```python
from build123d import *

# Parameters (mm, degrees)
SKETCH_1_R      = 1
SKETCH_1_W      = 5
SKETCH_1_H      = 2.8
EXTRUDE_1_DEPTH = 1.4


with BuildPart() as part:
    # Эскиз1 → Бобышка-Вытянуть1 (new, symmetric)
    with BuildSketch(Plane.XY):
        with BuildLine():
            ThreePointArc((223.382624747, 5.634990628), (219.398084745, 3.984540168), (217.747634119, 2.35e-07))
            ThreePointArc((217.747634119, 2.35e-07), (219.398084579, -3.984540002), (223.382624747, -5.634990628))
            add(Edge.make_bspline(
                [(223.382624746, -5.634990613), (224.328656864, -5.56201019), (226.923894547, -5.35916654), (231.150377303, -5.017351086), (234.870714804, -4.704112055), (236.94221324, -4.525459463), (237.382624747, -4.487285848)],
                knots=[0.670161589, 0.670161589, 0.670161589, 0.670161589, 0.686667237, 0.715444849, 0.743923546, 0.751613474, 0.751613474, 0.751613474, 0.751613474], degree=3))
            Line((237.382624747, -4.487285848), (241.902085906, -8.639702096))
            ThreePointArc((241.902085906, -8.639702096), (243.345073916, -9.164930306), (244.73509722, -8.51230922))
            Line((244.73509722, -8.51230922), (249.382624747, -3.400128388))
            add(Edge.make_bspline(
                [(249.382624747, -3.400128388), (251.158571989, -3.232274224), (254.371192488, -2.923000161), (258.952644662, -2.467188138), (263.047743378, -2.047856604), (266.898988862, -1.642607304), (270.455833183, -1.258590905), (273.651166984, -0.905304265), (276.385426802, -0.596436482), (278.45259621, -0.358958361), (279.592043704, -0.226075898), (280, -0.1785)],
                knots=[0.821480844, 0.821480844, 0.821480844, 0.821480844, 0.852512115, 0.877624446, 0.901571134, 0.924121062, 0.944988816, 0.963803939, 0.980044339, 0.992855276, 1, 1, 1, 1], degree=3))
            ThreePointArc((280, -0.1785), (280.073937121, 0), (280, 0.1785))
            add(Edge.make_bspline(
                [(280, 0.1785), (279.592043704, 0.226075898), (278.45259621, 0.358958361), (276.385426802, 0.596436482), (273.651166984, 0.905304265), (270.455833183, 1.258590905), (266.898988862, 1.642607304), (263.047743378, 2.047856604), (258.952644662, 2.467188138), (253.116111921, 3.047869044), (247.071089236, 3.62220531), (240.854179313, 4.184912649), (236.038226964, 4.605811749), (231.150377303, 5.017351103), (226.923894547, 5.359166556), (224.328656864, 5.562010205), (223.382624747, 5.634990628)],
                knots=[0, 0, 0, 0, 0.007144724, 0.019955661, 0.036196061, 0.055011184, 0.075878938, 0.098428866, 0.122375554, 0.147487885, 0.200459747, 0.22800517, 0.256076454, 0.284555151, 0.313332763, 0.329838411, 0.329838411, 0.329838411, 0.329838411], degree=3))
        make_face()
        with Locations((243.382624747, -6.903125596)):
            Circle(SKETCH_1_R, mode=Mode.SUBTRACT)
        with Locations((223.382624747, 0)):
            Circle(SKETCH_1_R, mode=Mode.SUBTRACT)
        with Locations((243.382624747, 0)):
            Rectangle(SKETCH_1_W, SKETCH_1_H, mode=Mode.SUBTRACT)
    extrude(amount=EXTRUDE_1_DEPTH, both=True)


solid = part.part
```
Here's how the part is built. I have some questions about the finished solid (model axes, mm). A direction names the side the tool comes from. Give positions to 0.01 mm unless a question says otherwise; leave off trailing zeros. Answer as a JSON object with one key per item and string values. Group by question number.
Item 1: For P1, Ø1, axis at x = 262, z = 0, coming from the +Y side; P2, Ø0.8, axis at y = 0.5, z = -0.5, coming from the +X side; P3, Ø0.8, axis at x = 242.5, z = 0.5, coming from the +Y side, each with a flat end and sliding along its axis, tell me the tip position at first contact or that it passes through.
Item 2: If we mould it in two halves opening along Y, with no side actions, what happens to faces 1 (the flat face through (243, 1.4, 0)), 2 (the flat face through (240.883, 0, 0)), 3 (the cylindrical face through (217.75, 0.12, 0.02)), 4 (the flat face through (247.03, -5.99, 0.02))? For each: pulls with the +Y half, pulls with the -Y half, needs draft (parallel to the pull), parting line crosses it, or undercut.
Item 3: If we section it at A-A on z = -0.45: Give the number of separate pieces and of enclosed holes in the cut face, and give its area (3 significant figures).
Item 4: Please list where these lines run through material, in increasing order: probe 1 along Y at (x, z) = (223.5, 1.2); probe 2 along X at (y, z) = (-7, 0.75); probe 3 along X at (y, z) = (-6.5, 0.45).
Item 5: Which directions (+Z, -Z, +X, -X, +Y, -Y) give clear straight access to the entire face, cutting with the end or side of a thin tool? Please do faces 5 (the flat face through (242, -2, 1.4)), 6 (the flat face through (245.883, 0, 0)), 7 (the flat face through (239.611, -6.534, 0.02)).
Result set:
{
 "1": {"P1": "y = 2.21", "P2": "x = 280.05", "P3": "y = 4.07"},
 "2": {"face 1": "undercut", "face 2": "undercut", "face 3": "parting line crosses it", "face 4": "pulls with the -Y half"},
 "3": {"separate pieces": "1", "enclosed holes": "3", "area": "415 mm²"},
 "4": {"probe 1": "-5.63 to -0.99, 0.99 to 5.63", "probe 2": "240.12 to 242.39, 244.38 to 246.11", "probe 3": "239.57 to 242.47, 244.3 to 246.56"},
 "5": {"face 5": "+Z, +X, -X, +Y, -Y", "face 6": "+Z, -Z", "face 7": "+Z, -Z, -Y"}
}
